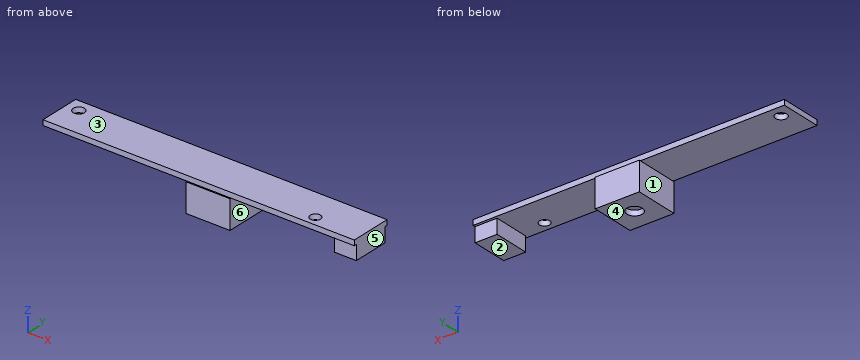
```python
from build123d import *

# Parameters (mm, degrees)
SKETCH_W        = 8.5
SKETCH_H        = 8.5
PAD_DEPTH       = 5.5
SKETCH001_W     = 60
SKETCH001_H     = 8
PAD001_DEPTH    = 1
SKETCH002_R     = 1
SKETCH002_R_2   = 1.1
POCKET_DEPTH    = 6.501
SKETCH003_W     = 4.25
SKETCH003_H     = 7
PAD002_DEPTH    = 2.8
SKETCH004_R     = 1.5
POCKET001_DEPTH = 1


with BuildPart() as part:
    # Sketch → Pad (new body)
    with BuildSketch(Plane.XY):
        Rectangle(SKETCH_W, SKETCH_H)
    extrude(amount=PAD_DEPTH)

    # Sketch001 → Pad001 (new body)
    with BuildSketch(Plane.XY.offset(5.5)):
        with Locations((-2, 0)):
            Rectangle(SKETCH001_W, SKETCH001_H)
    extrude(amount=PAD001_DEPTH)

    # Sketch002 → Pocket (cut, through all)
    with BuildSketch(Plane.XY.offset(6.5)):
        with Locations((19, -2.1)):
            Circle(SKETCH002_R)
        with Locations((-29.5, 1.6)):
            Circle(SKETCH002_R_2)
    extrude(amount=-POCKET_DEPTH, mode=Mode.SUBTRACT)

    # Sketch003 → Pad002 (new body)
    with BuildSketch(Plane(origin=(0, 0, 5.5), x_dir=(1, 0, 0), z_dir=(0, 0, -1))):
        with Locations((25.875, 0)):
            Rectangle(SKETCH003_W, SKETCH003_H)
    extrude(amount=PAD002_DEPTH)

    # Sketch004 → Pocket001 (cut)
    with BuildSketch(Plane(origin=(0, 0, 0), x_dir=(1, 0, 0), z_dir=(0, 0, -1))):
        Circle(SKETCH004_R)
    extrude(amount=-POCKET001_DEPTH, mode=Mode.SUBTRACT)


solid = part.part
```
The model under review builds one solid part; all positions refer to its coordinate system, in mm. Face numbers are marked on the shaded views. A direction names the side the tool comes from. Coordinates: 2 decimals unless noted, no trailing zeros. Write each loop counter-clockwise with the first axis right and the second up, starting at its lowest first coordinate (ties: lowest second). Pieces come first, ordered by that corner, then holes. Notation, with made-up numbers: (24.25, 36) -> (51.25, 36) arc R14 ccw to (51.25, 51) -> close; hole circle Ø10 at (-28, 41). An arc over 180 degrees is marked (long way). One line per item, written item: value. Start each with the question number.
Q1. Add section B-B, the plane z = 3.75. Give the boundary of the cut face in (x, y), then the cut area to 3 significant figures.
Q2. Add section A-A, the plane x = 19. Give the boundary of the cut face in (y, z), then the cut area to 3 significant figures.
Q3. To check wall thickness, follow probe 1 along Y at (x, z) = (-29.5, 5.8); probe 2 along Y at (x, z) = (0, 0.75); probe 3 along X at (y, z) = (-2, 5). State the ranges of each line that lie inside material, in increasing order.
Q4. For the marked faces 1, 2 and 3, list the 3-axis set-ups (+Z, -Z, +X, -X, +Y, -Y) from which the entire face can be reached by the end or side of a thin tool; tool diameter is ignored.
Q5. Add section C-C, the plane y = 0. Give the boundary of the cut face in (x, z).
Q6. Add section D-D, the plane x = 0. Give the boundary of the cut face in (y, z), then the cut area to 4 significant figures.
Q7. Clearance check with flat-ended pins moving along their axes: P1, Ø0.5, axis at x = -12, z = 6, coming from the -Y side; P2, Ø3, axis at x = 25.5, z = 3.5, coming from the -Y side; P3, Ø1.3, axis at x = 26.5, y = 0, coming from the -Z side; P4, Ø2, axis at y = 2, z = 2, coming from the +X side. State where each tip first meets the part, or that it passes through.
Q8. The part is to be moulded in two halves that separate along X. For the marked faces 4, 5 and 6, say which applies: +X half, -X half, draft (parallel to the pull), parting line (faces both ways), or undercut.
Response:
1. outline: (-4.25, -4.25) -> (4.25, -4.25) -> (4.25, 4.25) -> (-4.25, 4.25) -> close; (23.75, -3.5) -> (28, -3.5) -> (28, 3.5) -> (23.75, 3.5) -> close
1. area: 102 mm²
2. outline: (-4, 5.5) -> (-3.1, 5.5) -> (-3.1, 6.5) -> (-4, 6.5) -> close; (-1.1, 5.5) -> (4, 5.5) -> (4, 6.5) -> (-1.1, 6.5) -> close
2. area: 6.00 mm²
3. probe 1: -4 to 0.5, 2.7 to 4
3. probe 2: -4.25 to -1.5, 1.5 to 4.25
3. probe 3: -4.25 to 4.25, 23.75 to 28
4. face 1: -Z, -X, +Y, -Y
4. face 2: -Z, +X, +Y, -Y
4. face 3: +Z, +X, -X, +Y, -Y
5. outline: (-32, 5.5) -> (-4.25, 5.5) -> (-4.25, 0) -> (-1.5, 0) -> (-1.5, 1) -> (1.5, 1) -> (1.5, 0) -> (4.25, 0) -> (4.25, 5.5) -> (23.75, 5.5) -> (23.75, 2.7) -> (28, 2.7) -> (28, 6.5) -> (-32, 6.5) -> close
6. outline: (-4.25, 0) -> (-1.5, 0) -> (-1.5, 1) -> (1.5, 1) -> (1.5, 0) -> (4.25, 0) -> (4.25, 5.5) -> (4, 5.5) -> (4, 6.5) -> (-4, 6.5) -> (-4, 5.5) -> (-4.25, 5.5) -> close
6. area: 51.75 mm²
7. P1: y = -4
7. P2: y = -3.5
7. P3: z = 2.7
7. P4: x = 28
8. face 4: draft
8. face 5: +X half
8. face 6: undercut
